```python
from build123d import *
from build123d.topology import SkipClean

# Parameters (mm, degrees)
BOSS_EXTRUDE1_DEPTH = 4
SKETCH2_R           = 3
CUT_EXTRUDE1_DEPTH  = 2
SKETCH3_R           = 1.5
CUT_EXTRUDE2_DEPTH  = 22.633307653
CUT_EXTRUDE4_START  = -1.2
CUT_EXTRUDE4_DEPTH  = 1.2
CUT_EXTRUDE6_DEPTH  = 1.5
CUT_EXTRUDE7_DEPTH  = 0.7
BOSS_EXTRUDE3_DEPTH = 2
CUT_EXTRUDE12_START = -2
CUT_EXTRUDE12_DEPTH = 2
SKETCH6_R           = 2.5
CUT_EXTRUDE13_DEPTH = 22.777052142
SKETCH16_W          = 3
SKETCH16_H          = 5
BOSS_EXTRUDE4_DEPTH = 2
BOSS_EXTRUDE6_DEPTH = 1.9


with BuildPart() as part:
    # Sketch1 → Boss-Extrude1 (new body)
    with BuildSketch(Plane(origin=(0, 0, 0), x_dir=(1, 0, 0), z_dir=(0, 1, 0))):
        with BuildLine():
            Line((6.5, -20), (6.5, -4.663689527))
            ThreePointArc((6.5, -4.663689527), (7.615773106, -2.449489743), (8, 0))
            ThreePointArc((8, 0), (7.615773106, 2.449489743), (6.5, 4.663689527))
            ThreePointArc((6.5, 4.663689527), (0, 8), (-6.5, 4.663689527))
            ThreePointArc((-6.5, 4.663689527), (-7.615773106, 2.449489743), (-8, 0))
            ThreePointArc((-8, 0), (-7.615773106, -2.449489743), (-6.5, -4.663689527))
            Line((-6.5, -4.663689527), (-6.5, -20))
            Line((-6.5, -20), (6.5, -20))
        make_face()
    extrude(amount=BOSS_EXTRUDE1_DEPTH)

    # Sketch2 → Cut-Extrude1 (cut)
    with BuildSketch(Plane.XZ):
        with Locations(Location((0, 0, 0), (0, 0, 270))):
            Circle(SKETCH2_R)
    extrude(amount=-CUT_EXTRUDE1_DEPTH, mode=Mode.SUBTRACT)

    # Sketch3 → Cut-Extrude2 (cut, through all)
    with BuildSketch(Plane.XZ.offset(-2)):
        with Locations(Location((0, 0, 0), (0, 0, 270))):
            Circle(SKETCH3_R)
    extrude(amount=-CUT_EXTRUDE2_DEPTH, mode=Mode.SUBTRACT)

    # Sketch5 → Cut-Extrude4 (cut)
    with BuildSketch(Plane(origin=(0, 4, 0), x_dir=(1, 0, 0), z_dir=(0, 1, 0)).offset(CUT_EXTRUDE4_START)):
        with BuildLine():
            Line((5.75, 2.5), (2.5, 5.75))
            Line((2.5, 5.75), (0.75, 5.75))
            Line((0.75, 5.75), (0.75, 7.964766161))
            ThreePointArc((0.75, 7.964766161), (0, 8), (-0.75, 7.964766161))
            Line((-0.75, 7.964766161), (-0.75, 5.75))
            Line((-0.75, 5.75), (-2.5, 5.75))
            Line((-2.5, 5.75), (-5.75, 2.5))
            Line((-5.75, 2.5), (-5.75, -6.25))
            Line((-5.75, -6.25), (-4.4, -6.25))
            Line((-4.4, -6.25), (-4.4, -8.2))
            Line((-4.4, -8.2), (-5.66, -10))
            Line((-5.66, -10), (-6.5, -10))
            Line((-6.5, -10), (-6.5, -11.2))
            Line((-6.5, -11.2), (-6.5, -15))
            Line((-6.5, -15), (6.5, -15))
            Line((6.5, -15), (6.5, -11.2))
            Line((6.5, -11.2), (6.5, -10))
            Line((6.5, -10), (6.5, -8.2))
            Line((6.5, -8.2), (4.4, -8.2))
            Line((4.4, -8.2), (4.4, -6.25))
            Line((4.4, -6.25), (5.75, -6.25))
            Line((5.75, -6.25), (5.75, 2.5))
        make_face()
    extrude(amount=CUT_EXTRUDE4_DEPTH, mode=Mode.SUBTRACT)

    # Sketch7 → Cut-Extrude6 (cut)
    with BuildSketch(Plane(origin=(0, 2.8, 0), x_dir=(1, 0, 0), z_dir=(0, 1, 0))):
        with BuildLine():
            Line((-4.999999999, -5.5), (-4.999999999, -6.25))
            Line((-4.999999999, -6.25), (-3.499999999, -6.25))
            Line((-3.499999999, -6.25), (-3.499999999, -5.5))
            ThreePointArc((-3.499999999, -5.5), (-4.249999999, -4.75), (-4.999999999, -5.5))
        make_face()
        with BuildLine():
            Line((3.500000001, -5.5), (3.500000001, -6.25))
            Line((3.500000001, -6.25), (5.000000001, -6.25))
            Line((5.000000001, -6.25), (5.000000001, -5.5))
            ThreePointArc((5.000000001, -5.5), (4.250000001, -4.75), (3.500000001, -5.5))
        make_face()
    extrude(amount=-CUT_EXTRUDE6_DEPTH, mode=Mode.SUBTRACT)

    # Sketch9 → Cut-Extrude7 (cut)
    with BuildSketch(Plane(origin=(0, 2.8, 0), x_dir=(1, 0, 0), z_dir=(0, 1, 0))):
        Polygon((-6.5, -15), (6.5, -15), (6.5, -8.2), (4.4, -8.2), (4.4, -6.2), (-4.4, -6.2), (-4.4, -8.2), (-5.66, -10), (-6.5, -10), align=None)
    extrude(amount=-CUT_EXTRUDE7_DEPTH, mode=Mode.SUBTRACT)

    # Sketch14 → Boss-Extrude3 (add)
    with SkipClean():  # the faces are left unmerged after this step: merging them gives an invalid solid
        with BuildSketch(Plane(origin=(0, 4, 0), x_dir=(1, 0, 0), z_dir=(0, 1, 0))):
            with BuildLine():
                Line((6.5, -4.663689527), (6.5, 2.5))
                Line((6.5, 2.5), (7.599342077, 2.5))
                ThreePointArc((7.599342077, 2.5), (7.907431546, -1.213476964), (6.5, -4.663689527))
            make_face()
            with BuildLine():
                Line((-6.5, -4.663689527), (-6.5, 2.5))
                Line((-6.5, 2.5), (-7.599342077, 2.5))
                ThreePointArc((-7.599342077, 2.5), (-7.907431546, -1.213476964), (-6.5, -4.663689527))
            make_face()
        extrude(amount=BOSS_EXTRUDE3_DEPTH)

    # Sketch15 → Cut-Extrude12 (cut)
    with SkipClean():  # the faces are left unmerged after this step: merging them gives an invalid solid
        with BuildSketch(Plane(origin=(0, 4, 0), x_dir=(1, 0, 0), z_dir=(0, 1, 0)).offset(CUT_EXTRUDE12_START)):
            with BuildLine():
                Line((2.5, 5.75), (-2.5, 5.75))
                Line((-2.5, 5.75), (-4.125, 4.125))
                Line((-4.125, 4.125), (-5.656854249, 5.656854249))
                ThreePointArc((-5.656854249, 5.656854249), (0, 8), (5.656854249, 5.656854249))
                Line((5.656854249, 5.656854249), (4.125, 4.125))
                Line((4.125, 4.125), (2.5, 5.75))
            make_face()
        extrude(amount=CUT_EXTRUDE12_DEPTH, mode=Mode.SUBTRACT)

    # Sketch6 → Cut-Extrude13 (cut, through all)
    with SkipClean():  # the faces are left unmerged after this step: merging them gives an invalid solid
        with BuildSketch(Plane(origin=(0, 2.8, 0), x_dir=(1, 0, 0), z_dir=(0, 1, 0))):
            with Locations(Location((0, 0, 0), (0, 0, 270))):
                Circle(SKETCH6_R)
        extrude(amount=-CUT_EXTRUDE13_DEPTH, mode=Mode.SUBTRACT)

    # Sketch16 → Boss-Extrude4 (add)
    with SkipClean():  # the faces are left unmerged after this step: merging them gives an invalid solid
        with BuildSketch(Plane(origin=(0, 4, 0), x_dir=(1, 0, 0), z_dir=(0, 1, 0))):
            with Locations((0, -17.5)):
                Rectangle(SKETCH16_W, SKETCH16_H)
        extrude(amount=BOSS_EXTRUDE4_DEPTH)

    # Sketch18 → Boss-Extrude6 (add)
    with SkipClean():  # the faces are left unmerged after this step: merging them gives an invalid solid
        with BuildSketch(Plane(origin=(0, 2.1, 0), x_dir=(1, 0, 0), z_dir=(0, 1, 0))):
            Polygon((-4.4, -8.2), (-5.66, -10), (-6.5, -10), (-6.5, -15), (-4.4, -15), align=None)
        extrude(amount=BOSS_EXTRUDE6_DEPTH)


solid = part.part
```
Geometry: final body of the model. Coordinates: model frame, mm. A direction names the side the tool comes from. Round coordinates to 2 decimals unless told otherwise and drop trailing zeros. Write each loop counter-clockwise with the first axis right and the second up, starting at its lowest first coordinate (ties: lowest second). Pieces come first, ordered by that corner, then holes. Notation, with made-up numbers: M -37,28 L 21,28 A33 cw 21,60 Z; hole C -21.75,59.5 d7. An arc over 180 degrees is marked long. Answer in a Markdown table with one row per item. Add a question column.
(1) Draft query along Z for faces 4 (the face through (5, 3, -5)), 5 (the face through (-2.44, 2.41, -0.54)), 6 (the face through (0, 6, 17)). Return one class per face: pulls with the +Z half, pulls with the -Z half, needs draft (parallel to the pull), parting line crosses it, or undercut.
(2) Contact query for flat-ended pins moving along their axis: pin 1 (3 mm diameter, centred on x = -5, z = 17, fed in from +Y); pin 2 (1 mm diameter, centred on y = 5.5, z = 16.5, fed in from -X); pin 3 (2.5 mm diameter, centred on x = -5, y = 3, fed in from -Z). Output: stop coordinate, or through.
(3) Cut plane A-A, the plane y = 0.8. Return the cut outline in (x, z).
(4) Cut plane C-C, the plane z = 9.75. Return the cut outline in (x, y).
(5) Reachability of faces 1 (the face through (1, 4, 15)), 2 (the face through (-6.5, 2, 12)), 3 (the face through (4, 1.3, 5)) from +Z, -Z, +X, -X, +Y, -Y: full face, straight path, thin tool, end or side. Return the list, or none.
(6) Ray query, L1, parallel to Z at x = -1.75, y = 2.65; L2, parallel to Z at x = -0.25, y = 2.3; L3, parallel to Y at x = 3.5, z = -3.5. Return the intervals inside material, ascending.
(7) Cut plane B-B, the plane x = 0. Return the cut outline in (y, z), then the cut area to 3 significant figures.
Established:
| question | item | result |
|---|---|---|
| 1 | face 4 | pulls with the -Z half |
| 1 | face 5 | undercut |
| 1 | face 6 | needs draft |
| 2 | pin 1 | y = 4 |
| 2 | pin 2 | x = -1.5 |
| 2 | pin 3 | z = -6.78 |
| 3 | outline | M -6.5,4.66 A8 ccw long 6.5,4.66 L 6.5,20 L -6.5,20 Z; hole C 0,0 d6 |
| 4 | outline | M -6.5,0 L 6.5,0 L 6.5,2.1 L -4.4,2.1 L -4.4,4 L -6.5,4 Z |
| 5 | face 1 | +X, +Y |
| 5 | face 2 | +Z, -X, +Y, -Y |
| 5 | face 3 | +Y |
| 6 | L1 | -5.75 to -1.79, 1.79 to 6.2, 15 to 20 |
| 6 | L2 | -5.75 to -2.49, 2.49 to 6.2, 15 to 20 |
| 6 | L3 | 0 to 2.8 |
| 7 | outline | M 0,-8 L 2,-8 L 2,-5.75 L 2.8,-5.75 L 2.8,-2.5 L 2,-2.5 L 2,-3 L 0,-3 Z; M 0,3 L 2,3 L 2,2.5 L 2.8,2.5 L 2.8,6.2 L 2.1,6.2 L 2.1,15 L 6,15 L 6,20 L 0,20 Z |
| 7 | area | 70.4 mm² |
